Job drawing, mm, ordinate dimensions from the low corner. One solid piece. Coordinates: 2 decimals unless noted, no trailing zeros. Order: outer loops, then holes, each group sorted by start corner. A loop starts at its lowest first (then second) coordinate and runs counter-clockwise, first axis right, second up. Notation, with made-up numbers: (83, -36.5) - (118, -36.5) arc R9 cw to (118, -30.5) - close; hole circle Ø11 at (-12, 12.5). An arc over 180 degrees is marked (long way). Write each question's results on one line, items separated by ' | '. Start each with the question number.
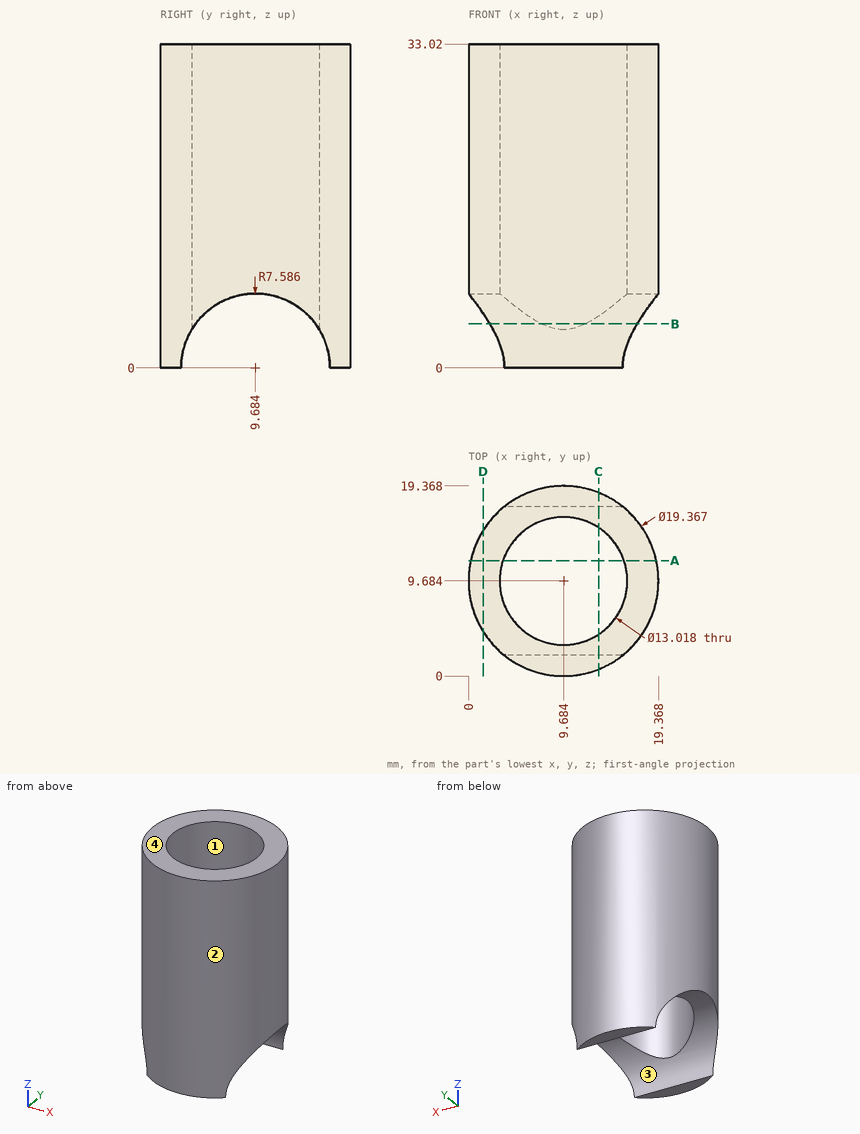
Item 1: Slice it at D-D (x = 1.5). Write the cut outline in (y, z) (1 decimal).
Item 2: Slice it at C-C (x = 13.25). Write the cut outline in (y, z) (1 decimal).
Item 3: Flat gauge pins, fed straight in: P1, Ø4, axis at y = 13, z = 19.5, coming from the -X side; P2, Ø3, axis at y = 4.5, z = 18.5, coming from the -X side; P3, Ø4, axis at x = 15, z = 21, coming from the -Y side (1 decimal); P4, Ø3, axis at x = 9.5, y = 13.5, coming from the +Z side. Where does each tip first touch, or does it go through?
Item 4: Probe probe 1 along X at (y, z) = (9.5, 11) (1 decimal); probe 2 along Y at (x, z) = (7.25, 4.5) (1 decimal); probe 3 along Y at (x, z) = (15.5, 23.5) (1 decimal). List the from-to ranges inside material, lowest first.
Item 5: Slice it at B-B (z = 4.5). Write the cut outline in (x, y) (1 decimal).
Item 6: Pull direction Y, two halves, no side cores. Call the marked faces 1, 2, 3 and 4: released by +Y, released by -Y, zero draft, split by the parting line, or undercut.
Item 7: Slice it at A-A (y = 11.75). Write the cut outline in (x, z) (1 decimal), then the cut area to 3 significant figures.
Resolved:
1) outline: (4.5, 5.5) arc R7.6 cw to (14.9, 5.5) - (14.9, 33) - (4.5, 33) - close
2) outline: (0.7, 0) - (2.1, 0) arc R7.6 cw to (4.2, 5.3) - (4.2, 33) - (0.7, 33) - close; (15.1, 5.3) arc R7.6 cw to (17.3, 0) - (18.7, 0) - (18.7, 33) - (15.1, 33) - close
3) P1: x = 0.09 | P2: x = 0.73 | P3: y = 0.6 | P4: through
4) probe 1: 0 to 3.2, 16.2 to 19.4 | probe 2: 0.3 to 3.6, 15.8 to 19.1 | probe 3: 1.9 to 6.8, 12.6 to 17.4
5) outline: (2.2, 3.6) arc R9.7 ccw to (17.2, 3.6) - (11.9, 3.6) arc R6.5 cw to (7.4, 3.6) - close; (2.2, 15.8) - (7.4, 15.8) arc R6.5 cw to (11.9, 15.8) - (17.2, 15.8) arc R9.7 ccw to start
6) face 1: undercut | face 2: split by the parting line | face 3: undercut | face 4: zero draft
7) outline: (0.2, 7.3) - (3.5, 7.3) - (3.5, 33) - (0.2, 33) - close; (15.9, 7.3) - (19.1, 7.3) - (19.1, 33) - (15.9, 33) - close | area: 169 mm^2
